from build123d import *

# Parameters (mm, degrees)
CROQUIS1_W                 = 76.2
CROQUIS1_H                 = 76.2
SALIENTE_EXTRUIR1_DEPTH    = 2600
SALIENTE_EXTRUIR1_2_DEPTH  = 2600
SALIENTE_EXTRUIR1_3_DEPTH  = 2600
SALIENTE_EXTRUIR1_4_DEPTH  = 2600
SALIENTE_EXTRUIR1_5_DEPTH  = 2600
SALIENTE_EXTRUIR1_6_DEPTH  = 2600
SALIENTE_EXTRUIR1_7_DEPTH  = 2600
SALIENTE_EXTRUIR1_8_DEPTH  = 2600
SALIENTE_EXTRUIR1_9_DEPTH  = 2600
SALIENTE_EXTRUIR1_10_DEPTH = 2600
CROQUIS2_W                 = 76.2
CROQUIS2_H                 = 76.2
SALIENTE_EXTRUIR2_DEPTH    = 1100
CROQUIS3_W                 = 1252.4
CROQUIS3_H                 = 2600
CORTAR_EXTRUIR1_DEPTH      = 5924.8


with BuildPart() as part:
    # Croquis1 → Saliente-Extruir1 (new body)
    with BuildSketch(Plane(origin=(0, 0, 0), x_dir=(1, 0, 0), z_dir=(0, 1, 0))):
        with Locations((38.1, -38.1)):
            Rectangle(CROQUIS1_W, CROQUIS1_H)
    extrude(amount=SALIENTE_EXTRUIR1_DEPTH)



with BuildPart() as body_2:
    # Croquis1 → Saliente-Extruir1 2 (new body)
    with BuildSketch(Plane(origin=(0, 0, 0), x_dir=(1, 0, 0), z_dir=(0, 1, 0))):
        with Locations((1519.3, -38.1)):
            Rectangle(CROQUIS1_W, CROQUIS1_H)
    extrude(amount=SALIENTE_EXTRUIR1_2_DEPTH)


with BuildPart() as body_3:
    # Croquis1 → Saliente-Extruir1 3 (new body)
    with BuildSketch(Plane(origin=(0, 0, 0), x_dir=(1, 0, 0), z_dir=(0, 1, 0))):
        with Locations((3000.5, -38.1)):
            Rectangle(CROQUIS1_W, CROQUIS1_H)
    extrude(amount=SALIENTE_EXTRUIR1_3_DEPTH)


with BuildPart() as body_4:
    # Croquis1 → Saliente-Extruir1 4 (new body)
    with BuildSketch(Plane(origin=(0, 0, 0), x_dir=(1, 0, 0), z_dir=(0, 1, 0))):
        with Locations((4481.7, -38.1)):
            Rectangle(CROQUIS1_W, CROQUIS1_H)
    extrude(amount=SALIENTE_EXTRUIR1_4_DEPTH)


with BuildPart() as body_5:
    # Croquis1 → Saliente-Extruir1 5 (new body)
    with BuildSketch(Plane(origin=(0, 0, 0), x_dir=(1, 0, 0), z_dir=(0, 1, 0))):
        with Locations((5962.9, -38.1)):
            Rectangle(CROQUIS1_W, CROQUIS1_H)
    extrude(amount=SALIENTE_EXTRUIR1_5_DEPTH)


with BuildPart() as body_6:
    # Croquis1 → Saliente-Extruir1 6 (new body)
    with BuildSketch(Plane(origin=(0, 0, 0), x_dir=(1, 0, 0), z_dir=(0, 1, 0))):
        with Locations((5962.9, -1214.3)):
            Rectangle(CROQUIS1_W, CROQUIS1_H)
    extrude(amount=SALIENTE_EXTRUIR1_6_DEPTH)


with BuildPart() as body_7:
    # Croquis1 → Saliente-Extruir1 7 (new body)
    with BuildSketch(Plane(origin=(0, 0, 0), x_dir=(1, 0, 0), z_dir=(0, 1, 0))):
        with Locations((4481.7, -1214.3)):
            Rectangle(CROQUIS1_W, CROQUIS1_H)
    extrude(amount=SALIENTE_EXTRUIR1_7_DEPTH)


with BuildPart() as body_8:
    # Croquis1 → Saliente-Extruir1 8 (new body)
    with BuildSketch(Plane(origin=(0, 0, 0), x_dir=(1, 0, 0), z_dir=(0, 1, 0))):
        with Locations((3000.5, -1214.3)):
            Rectangle(CROQUIS1_W, CROQUIS1_H)
    extrude(amount=SALIENTE_EXTRUIR1_8_DEPTH)


with BuildPart() as body_9:
    # Croquis1 → Saliente-Extruir1 9 (new body)
    with BuildSketch(Plane(origin=(0, 0, 0), x_dir=(1, 0, 0), z_dir=(0, 1, 0))):
        with Locations((1519.3, -1214.3)):
            Rectangle(CROQUIS1_W, CROQUIS1_H)
    extrude(amount=SALIENTE_EXTRUIR1_9_DEPTH)


with BuildPart() as body_10:
    # Croquis1 → Saliente-Extruir1 10 (new body)
    with BuildSketch(Plane(origin=(0, 0, 0), x_dir=(1, 0, 0), z_dir=(0, 1, 0))):
        with Locations((38.1, -1214.3)):
            Rectangle(CROQUIS1_W, CROQUIS1_H)
    extrude(amount=SALIENTE_EXTRUIR1_10_DEPTH)


with BuildPart() as part_1:
    add(part.part)

    add(body_2.part)  # Saliente-Extruir2 merges body 2

    add(body_3.part)  # Saliente-Extruir2 merges body 3

    add(body_4.part)  # Saliente-Extruir2 merges body 4

    add(body_5.part)  # Saliente-Extruir2 merges body 5

    add(body_6.part)  # Saliente-Extruir2 merges body 6

    add(body_7.part)  # Saliente-Extruir2 merges body 7

    add(body_8.part)  # Saliente-Extruir2 merges body 8

    add(body_9.part)  # Saliente-Extruir2 merges body 9

    add(body_10.part)  # Saliente-Extruir2 merges body 10
    # Croquis2 → Saliente-Extruir2 (add)
    with BuildSketch(Plane.XY.offset(76.2)):
        with Locations((38.1, 2561.9)):
            Rectangle(CROQUIS2_W, CROQUIS2_H)
        with Locations((1519.3, 2561.9)):
            Rectangle(CROQUIS2_W, CROQUIS2_H)
        with Locations((3000.5, 2561.9)):
            Rectangle(CROQUIS2_W, CROQUIS2_H)
        with Locations((4481.7, 2561.9)):
            Rectangle(CROQUIS2_W, CROQUIS2_H)
        with Locations((5962.9, 2561.9)):
            Rectangle(CROQUIS2_W, CROQUIS2_H)
    extrude(amount=SALIENTE_EXTRUIR2_DEPTH)

    # Croquis3 → Cortar-Extruir1 (cut)
    with BuildSketch(Plane(origin=(6001, 0, 0), x_dir=(0, 0, -1), z_dir=(1, 0, 0))):
        with Locations((-626.2, 1300)):
            Rectangle(CROQUIS3_W, CROQUIS3_H)
    extrude(amount=-CORTAR_EXTRUIR1_DEPTH, mode=Mode.SUBTRACT)


solid = part_1.part
Source: CAD feature listing. Evaluate the final solid. Frame: model axes, mm. A direction names the side the tool comes from. Coordinates: 2 decimals unless noted, no trailing zeros. Order: outer loops, then holes, each group sorted by start corner. A loop starts at its lowest first (then second) coordinate and runs counter-clockwise, first axis right, second up.
Item 1: Cut plane C-C (z = 521.5). Return loops of the section in (x, y).
Output values:
outline: (0, 2523.8) - (76.2, 2523.8) - (76.2, 2600) - (0, 2600) - close
Item 2: Set-up query: faces 1 (the face through (38, 1282, 0)), 2 (the face through (38, 2523.8, 618)). Return all of +Z, -Z, +X, -X, +Y, -Y with unobstructed straight access to the full face (end or side cutting, diameter ignored); none if empty.
Output values:
face 1: -Z, +X, -X, +Y, -Y
face 2: +X, -X, -Y
Item 3: Cut plane A-A (y = 424). Return loops of the section in (x, z).
Output values:
outline: (0, 0) - (76.2, 0) - (76.2, 76.2) - (0, 76.2) - close; (0, 1176.2) - (76.2, 1176.2) - (76.2, 1252.4) - (0, 1252.4) - close
Item 4: Material intervals for line 1 (Z direction, x = 61.5, y = 758.5); line 2 (Y direction, x = 58.5, z = 110.5), sorted ascending.
Output values:
line 1: z = 0 to 76.2, 1176.2 to 1252.4
line 2: y = 2523.8 to 2600
Item 5: Pull-direction query (Z, two-part tool) for faces 3 (the face through (38, 0, 38)), 4 (the face through (38, 1244, 76.2)), 5 (the face through (38, 1282, 1252.4)); classes: pulls with the +Z half, pulls with the -Z half, needs draft (parallel to the pull), parting line crosses it, or undercut.
Output values:
face 3: needs draft
face 4: undercut
face 5: pulls with the +Z half
Item 6: Cut plane B-B (x = 22). Return loops of the section in (y, z), plus the area to 3 significant figures.
Output values:
outline: (0, 0) - (2600, 0) - (2600, 1252.4) - (0, 1252.4) - (0, 1176.2) - (2523.8, 1176.2) - (2523.8, 76.2) - (0, 76.2) - close
area: 480,000 mm2
